Verification items for this drawing (mm, ordinates from the low corner). A direction names the side the tool comes from. Give positions to 0.01 mm unless a question says otherwise; leave off trailing zeros. Loops run counter-clockwise (first coordinate to the right, second up) from the corner with the lowest first, then second, coordinate; pieces in that order, holes last. Notation, with made-up numbers: (33.25, -23) -> (43.25, -23) arc R15 ccw to (43.25, -18) -> close; hole circle Ø5 at (19, -31.5). An arc over 180 degrees is marked (long way). Answer as a JSON object with one key per item and string values.
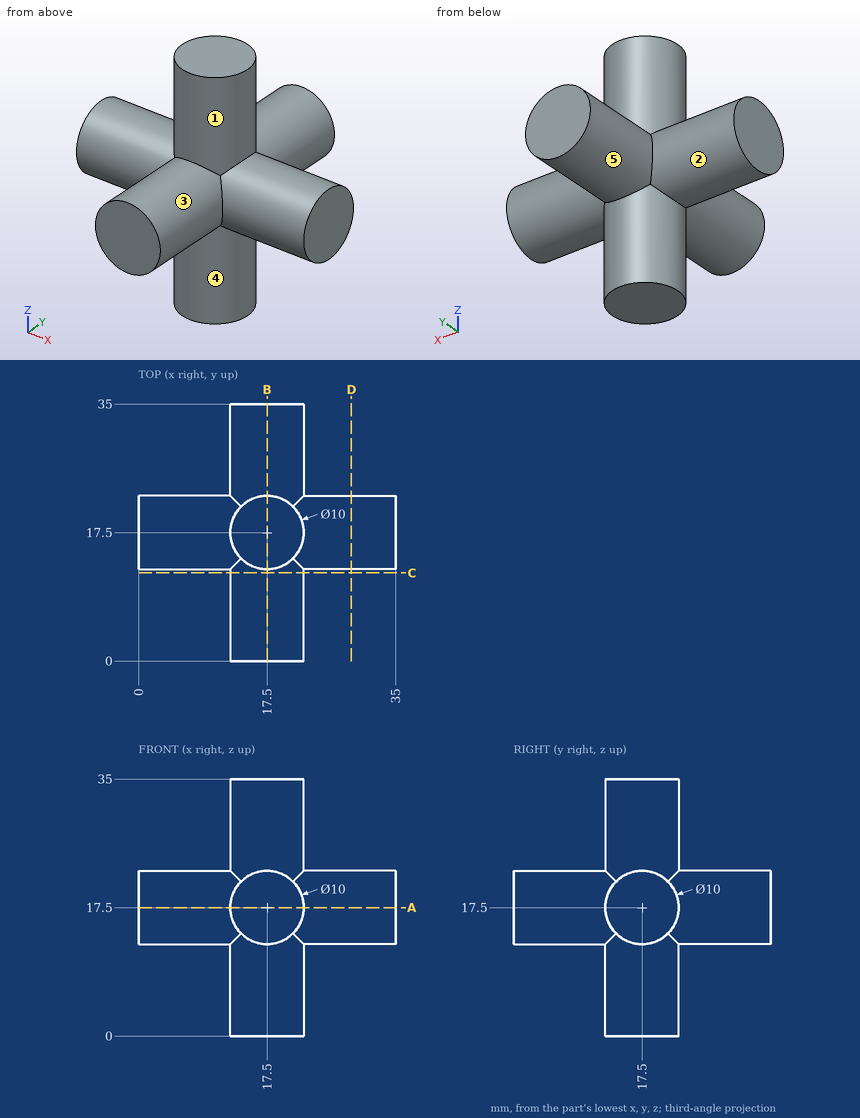
1) Section check A-A on z = 17.5. Record the cut outline in (x, y), plus the area to 3 significant figures.
Geometry check:
{"outline": "(0, 12.5) -> (12.5, 12.5) -> (12.5, 0) -> (22.5, 0) -> (22.5, 12.5) -> (35, 12.5) -> (35, 22.5) -> (22.5, 22.5) -> (22.5, 35) -> (12.5, 35) -> (12.5, 22.5) -> (0, 22.5) -> close", "area": "600 mm2"}
2) Tool access check on the marked faces 1, 2, 3, 4 and 5. Record the directions out of +Z, -Z, +X, -X, +Y, -Y that give a thin tool (end or side, any length) a straight path to the whole face; none if there is none.
Geometry check:
{"face 1": "+Z", "face 2": "-X", "face 3": "-Y", "face 4": "-Z", "face 5": "+Y"}
3) Section check C-C on y = 12. Record the cut outline in (x, z), plus the area to 3 significant figures.
Geometry check:
{"outline": "circle Ø10 at (17.5, 17.5)", "area": "78.5 mm2"}
4) Depth check by flat-ended pin: P1, Ø5, axis at x = 14, y = 26, coming from the -Z side; P2, Ø1.5, axis at x = 17, y = 12.5, coming from the -Z side; P3, Ø10, axis at x = 22, y = 28.5, coming from the +Z side; P4, Ø4, axis at y = 6.5, z = 10, coming from the -X side. Enter the tip coordinate at first touch or a pass-through.
Geometry check:
{"P1": "stops at z = 12.6", "P2": "stops at z = 0", "P3": "stops at z = 22.5", "P4": "passes through"}
5) Material ranges on line 1 along Z through (x, y) = (3.5, 14.5); line 2 along Y through (x, z) = (3, 14); line 3 along Z through (x, y) = (10.5, 21.5), recorded low to high. Write a range as from..to.
Geometry check:
{"line 1": "z = 13.5..21.5", "line 2": "y = 13.93..21.07", "line 3": "z = 14.5..20.5"}
